The figure shows three views and two pictorial views of one solid part (mm, origin at its lowest corner). Answer the questions. A direction names the side the tool comes from. Round coordinates to 2 decimals unless told otherwise and drop trailing zeros. Order: outer loops, then holes, each group sorted by start corner. A loop starts at its lowest first (then second) coordinate and runs counter-clockwise, first axis right, second up. Notation, with made-up numbers: (48.5, 2) - (82.5, 2) arc R23 ccw to (82.5, 24) - close; hole circle Ø7 at (10, -29.5). An arc over 180 degrees is marked (long way). Answer as a JSON object with one key per item and string values. Group by question number.
Q1. A cutting plane is placed at C-C on y = 56. Determine the outline of the cut face in (x, z).
Q2. A cutting plane is placed at A-A on z = 17. Determine the outline of the cut face in (x, y).
Q3. A tool of negligible diameter and unlimited length cuts with its end or side. For the marked faces 1, 2, 3, 4 and 5, from which of +Z, -Z, +X, -X, +Y, -Y can it reach the whole face along a straight path? Write none if from no direction.
Q4. A cutting plane is placed at B-B on x = 50. Determine the outline of the cut face in (y, z), and give its area (3 significant figures).
Q5. Consider line 1 (X direction, y = 9.5, z = 51); line 2 (X direction, y = 21, z = 18); line 3 (Y direction, x = 24.5, z = 3.5). Determine where each line is inside the solid, lowest interval first.
Q6. A cutting plane is placed at D-D on x = 4. Determine the outline of the cut face in (y, z).
Q7. Given pin 1 Ø16 at (x, y) = (52.5, 53) entering from +Z; pin 2 Ø22 at (y, z) = (8.5, 35) entering from -X; pin 3 Ø12 at (x, z) = (21, 20) entering from +Y; pin 4 Ø1.5 at (x, z) = (22, 35.5) entering from -Y, each flat-ended and moving along its own axis, determine where each tip first touches the part or whether it passes through.
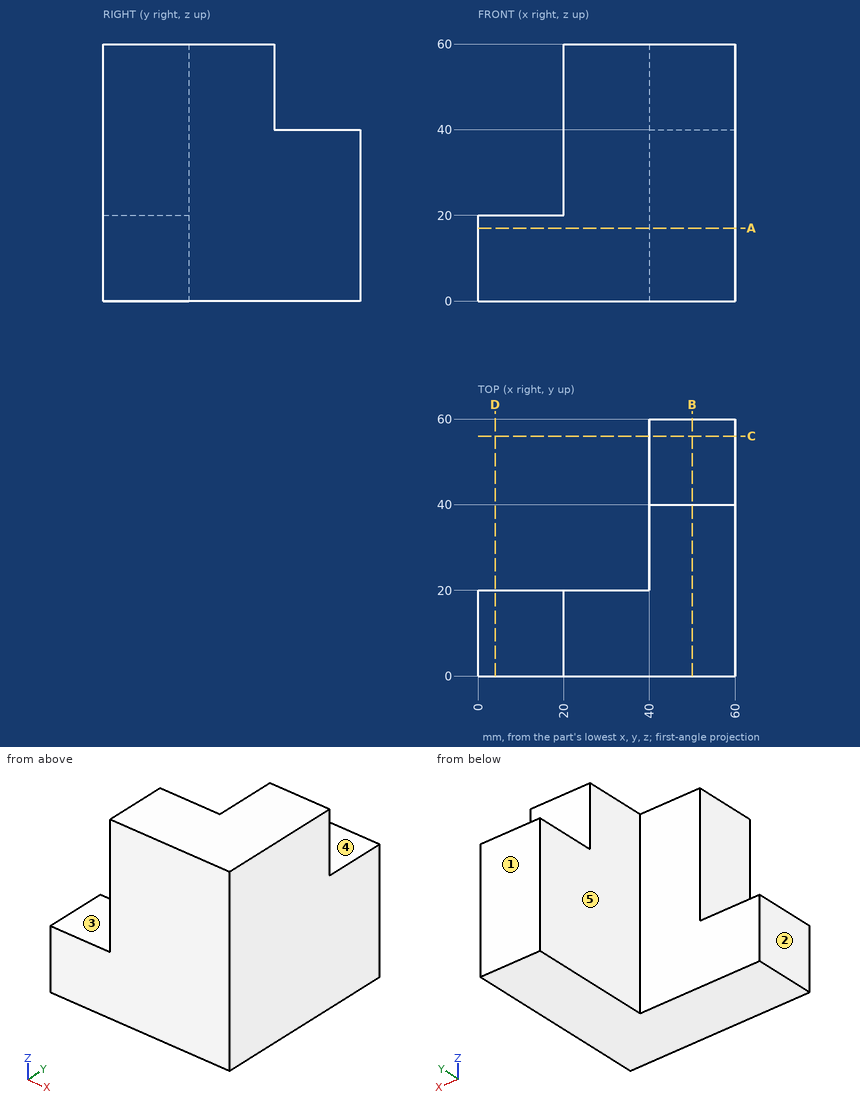
Result set:
{
 "1": {"outline": "(40, 0) - (60, 0) - (60, 40) - (40, 40) - close"},
 "2": {"outline": "(0, 0) - (60, 0) - (60, 60) - (40, 60) - (40, 20) - (0, 20) - close"},
 "3": {"face 1": "+Z, -Z, +X, -X, +Y", "face 2": "+Z, -Z, -X, +Y, -Y", "face 3": "+Z, -X, +Y, -Y", "face 4": "+Z, +X, -X, +Y", "face 5": "+Z, -Z, -X, +Y"},
 "4": {"outline": "(0, 0) - (60, 0) - (60, 40) - (40, 40) - (40, 60) - (0, 60) - close", "area": "3,200 mm²"},
 "5": {"line 1": "x = 20 to 60", "line 2": "x = 40 to 60", "line 3": "y = 0 to 20"},
 "6": {"outline": "(0, 0) - (20, 0) - (20, 20) - (0, 20) - close"},
 "7": {"pin 1": "stops at z = 40", "pin 2": "stops at x = 20", "pin 3": "stops at y = 20", "pin 4": "stops at y = 0"}
}
